The listing builds one solid part. Answer for the finished solid, in the listing's coordinates (mm). Round coordinates to 2 decimals unless told otherwise and drop trailing zeros. Order: outer loops, then holes, each group sorted by start corner. A loop starts at its lowest first (then second) coordinate and runs counter-clockwise, first axis right, second up. Notation, with made-up numbers: (-2, 26.5) -> (2, 26.5) arc R18 ccw to (2, 58.5) -> close; hole circle Ø4 at (-24.75, 57.25). An arc over 180 degrees is marked (long way). Answer in a Markdown table with one row per item. Add a question column.
```python
from build123d import *

# Parameters (mm, degrees)
F0_R     = 1.75
F1_DEPTH = 3
F2_SIZE2 = 2.8
F2_SIZE  = 1.6
F4_DEPTH = 0.5
F5_SIZE  = 0.49999
F7_DEPTH = 0.2


# Not quite as in the source:
# - a fillet or chamfer is up to 0.001 mm smaller than in the source, because OpenCascade refuses the exact size


with BuildPart() as f1:
    # F0 (on Top) → F1 (new body)
    with BuildSketch(Plane.XY):
        with BuildLine():
            Line((18.2, -38.893), (18.2, -44.793))
            ThreePointArc((18.2, -44.793), (22.9, -49.493), (27.6, -44.793))
            Line((27.6, -44.793), (27.6, -38.893))
            Line((27.6, -38.893), (39.8048274606, -38.893))
            Line((39.8048274606, -38.893), (50.3215900894, -49.3928583233))
            Line((50.3215900894, -49.3928583233), (68.3003446043, -49.3928583233))
            Line((68.3003446043, -49.3928583233), (68.3003446043, 33.6071416767))
            ThreePointArc((68.3003446043, 33.6071416767), (63.6003446043, 38.3071416767), (58.9003446043, 33.6071416767))
            Line((58.9003446043, 33.6071416767), (58.9003446043, 27.7071416767))
            Line((58.9003446043, 27.7071416767), (-0.4976553957, 27.7071416767))
            Line((-0.4976553957, 27.7071416767), (-0.4976553957, 33.6071416767))
            ThreePointArc((-0.4976553957, 33.6071416767), (-5.1976553957, 38.3071416767), (-9.8976553957, 33.6071416767))
            Line((-9.8976553957, 33.6071416767), (-9.8976553957, 10.7295926865))
            Line((-9.8976553957, 10.7295926865), (0.6, 0.248810884))
            Line((0.6, 0.248810884), (0.6, -38.893))
            Line((0.6, -38.893), (18.2, -38.893))
        make_face()
        with Locations((22.9, -44.793)):
            Circle(F0_R, mode=Mode.SUBTRACT)
        with Locations((-5.1976553957, 33.6071416767)):
            Circle(F0_R, mode=Mode.SUBTRACT)
        with Locations((63.6003446043, 33.6071416767)):
            Circle(F0_R, mode=Mode.SUBTRACT)
    extrude(amount=F1_DEPTH)

    # F2
    f2_edges = [f1.edges().sort_by_distance(p)[0] for p in [
        (21.15, -44.793, 0),
        (-6.947655, 33.607142, 0),
        (61.850345, 33.607142, 0),
    ]]
    f2_side = f1.faces().sort_by_distance((33.412828, -5.806914, 0))[0]
    chamfer(f2_edges, length=F2_SIZE, length2=F2_SIZE2, reference=f2_side)

    # F3 (on face) → F4 (cut)
    with BuildSketch(Plane.XY.offset(3)):
        with BuildLine():
            Line((-9.8976553957, 27.7071416767), (-0.4976553957, 27.7071416767))
            Line((-0.4976553957, 27.7071416767), (-0.4976553957, 33.6071416767))
            ThreePointArc((-0.4976553957, 33.6071416767), (-5.1976553957, 38.3071416767), (-9.8976553957, 33.6071416767))
            Line((-9.8976553957, 33.6071416767), (-9.8976553957, 27.7071416767))
        make_face()
        with BuildLine():
            Line((58.9003446043, 33.6071416767), (58.9003446043, 27.7071416767))
            Line((58.9003446043, 27.7071416767), (68.3003446043, 27.7071416767))
            Line((68.3003446043, 27.7071416767), (68.3003446043, 33.6071416767))
            ThreePointArc((68.3003446043, 33.6071416767), (63.6003446043, 38.3071416767), (58.9003446043, 33.6071416767))
        make_face()
        with BuildLine():
            Line((27.6, -38.893), (18.2, -38.893))
            Line((18.2, -38.893), (18.2, -44.793))
            ThreePointArc((18.2, -44.793), (22.9, -49.493), (27.6, -44.793))
            Line((27.6, -44.793), (27.6, -38.893))
        make_face()
    extrude(amount=-F4_DEPTH, mode=Mode.SUBTRACT)

    # F5 (size 0.5 in the source; OpenCascade refuses exactly that, so slightly less here)
    f5_edges = [f1.edges().sort_by_distance(p)[0] for p in [
        (29.201345, 27.707142, 3),
        (-9.897655, 19.218367, 3),
        (-4.648828, 5.489202, 3),
        (0.6, -19.322095, 3),
        (20.202414, -38.893, 3),
        (45.063209, -44.142929, 3),
        (59.310967, -49.392858, 3),
        (68.300345, -10.842858, 3),
    ]]
    chamfer(f5_edges, length=F5_SIZE)

    # F6 (on face) → F7 (join)
    with BuildSketch(Plane(origin=(0, 0, 0), x_dir=(1, 0, 0), z_dir=(0, 0, -1))):
        with BuildLine():
            ThreePointArc((0.6, 43.893), (-2.9355339059, 42.4285339059), (-4.4, 38.893))
            Line((-4.4, 38.893), (-4.4, 1.824613149))
            Line((-4.4, 1.824613149), (-13.4303444218, -7.1912161881))
            ThreePointArc((-13.4303444218, -7.1912161881), (-14.5162831751, -8.8143179191), (-14.8976553957, -10.7295926865))
            Line((-14.8976553957, -10.7295926865), (-14.8976553957, -33.6071416767))
            ThreePointArc((-14.8976553957, -33.6071416767), (-5.1976553957, -43.3071416767), (4.5023446043, -33.6071416767))
            Line((4.5023446043, -33.6071416767), (4.5023446043, -32.7071416767))
            Line((4.5023446043, -32.7071416767), (53.9003446043, -32.7071416767))
            Line((53.9003446043, -32.7071416767), (53.9003446043, -33.6071416767))
            ThreePointArc((53.9003446043, -33.6071416767), (63.6003446043, -43.3071416767), (73.3003446043, -33.6071416767))
            Line((73.3003446043, -33.6071416767), (73.3003446043, 49.3928583233))
            ThreePointArc((73.3003446043, 49.3928583233), (71.8358785102, 52.9283922293), (68.3003446043, 54.3928583233))
            Line((68.3003446043, 54.3928583233), (50.3215900894, 54.3928583233))
            ThreePointArc((50.3215900894, 54.3928583233), (48.4100308427, 54.0130251219), (46.7889010633, 52.9312348218))
            Line((46.7889010633, 52.9312348218), (37.736115085, 43.893))
            Line((37.736115085, 43.893), (32.6, 43.893))
            Line((32.6, 43.893), (32.6, 44.793))
            ThreePointArc((32.6, 44.793), (22.9, 54.493), (13.2, 44.793))
            Line((13.2, 44.793), (13.2, 43.893))
            Line((13.2, 43.893), (0.6, 43.893))
        make_face()
        with BuildLine():
            Line((-9.8976553957, -33.6071416767), (-9.8976553957, -10.7295926865))
            Line((-9.8976553957, -10.7295926865), (0.6, -0.248810884))
            Line((0.6, -0.248810884), (0.6, 38.893))
            Line((0.6, 38.893), (18.2, 38.893))
            Line((18.2, 38.893), (18.2, 44.793))
            ThreePointArc((18.2, 44.793), (22.9, 49.493), (27.6, 44.793))
            Line((27.6, 44.793), (27.6, 38.893))
            Line((27.6, 38.893), (39.8048274606, 38.893))
            Line((39.8048274606, 38.893), (50.3215900894, 49.3928583233))
            Line((50.3215900894, 49.3928583233), (68.3003446043, 49.3928583233))
            Line((68.3003446043, 49.3928583233), (68.3003446043, -33.6071416767))
            ThreePointArc((68.3003446043, -33.6071416767), (63.6003446043, -38.3071416767), (58.9003446043, -33.6071416767))
            Line((58.9003446043, -33.6071416767), (58.9003446043, -27.7071416767))
            Line((58.9003446043, -27.7071416767), (-0.4976553957, -27.7071416767))
            Line((-0.4976553957, -27.7071416767), (-0.4976553957, -33.6071416767))
            ThreePointArc((-0.4976553957, -33.6071416767), (-5.1976553957, -38.3071416767), (-9.8976553957, -33.6071416767))
        make_face(mode=Mode.SUBTRACT)
    extrude(amount=-F7_DEPTH)


solid = f1.part
```
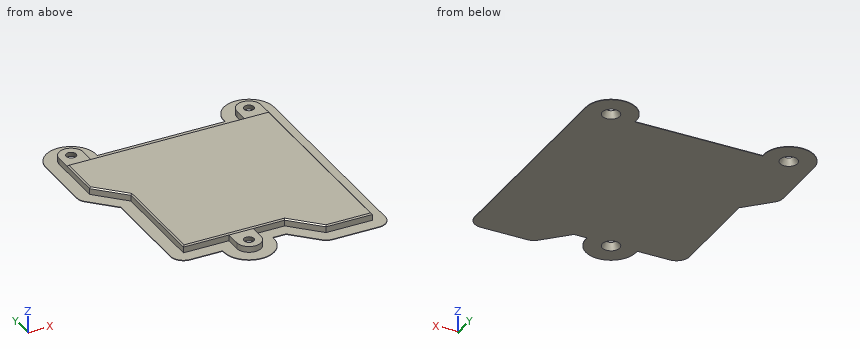
1. The part is cut by section B-B (x = 8). Give the vertices of the cut face in (y, z), then the cut area to 3 significant figures.
2. Each of these flat-tipped pins is pushed along its axis until it touches: pin 1 (4.5 mm diameter, centred on x = 22, y = -44.5, fed in from +Z); pin 2 (6 mm diameter, centred on x = 36.5, y = -44.5, fed in from -Z); pin 3 (3 mm diameter, centred on x = 11, y = -42, fed in from +Z); pin 4 (1.2 mm diameter, centred on x = 33.5, z = 2, fed in from +Y). Where does it stop, or does it pass through?
3. The part is cut by section A-A (z = 1.9). Give the vertices of the cut face in (x, y), then the cut area to 3 significant figures.
4. The part is cut by section C-C (y = -15.5). Give the vertices of the cut face in (x, z).
5. Straight lines are drawn through the part: line 1 along X through (y, z) = (32, 0.45); line 2 along Z through (x, y) = (69, 32.5); line 3 along Y through (x, z) = (9.5, 2.2). For each, find the intervals that lie inside material, in ascending order.
Report:
| question | item | result |
|---|---|---|
| 1 | outline | (-43.89, 0) -> (32.71, 0) -> (32.71, 0.2) -> (27.71, 0.2) -> (27.71, 2.5) -> (27.21, 3) -> (-38.39, 3) -> (-38.89, 2.5) -> (-38.89, 0.2) -> (-43.89, 0.2) -> close |
| 1 | area | 202 mm^2 |
| 2 | pin 1 | stops at z = 2.5 |
| 2 | pin 2 | stops at z = 0 |
| 2 | pin 3 | stops at z = 0.2 |
| 2 | pin 4 | stops at y = 27.71 |
| 3 | outline | (-9.9, 10.73) -> (0.6, 0.25) -> (0.6, -38.89) -> (18.2, -38.89) -> (18.2, -44.79) arc R4.7 ccw to (27.6, -44.79) -> (27.6, -38.89) -> (39.8, -38.89) -> (50.32, -49.39) -> (68.3, -49.39) -> (68.3, 33.61) arc R4.7 ccw to (58.9, 33.61) -> (58.9, 27.71) -> (-0.5, 27.71) -> (-0.5, 33.61) arc R4.7 ccw to (-9.9, 33.61) -> close; hole circle Ø4.53 at (-5.2, 33.61); hole circle Ø4.53 at (22.9, -44.79); hole circle Ø4.53 at (63.6, 33.61) |
| 3 | area | 5,210 mm^2 |
| 4 | outline | (-4.4, 0) -> (73.3, 0) -> (73.3, 0.2) -> (68.3, 0.2) -> (68.3, 2.5) -> (67.8, 3) -> (1.1, 3) -> (0.6, 2.5) -> (0.6, 0.2) -> (-4.4, 0.2) -> close |
| 5 | line 1 | x = -9.9 to -7.84, -2.56 to -0.5, 58.9 to 60.96, 66.24 to 68.3 |
| 5 | line 2 | z = 0 to 0.2 |
| 5 | line 3 | y = -38.89 to 27.71 |
